Design review of the part built by this model. Coordinates are the model's own, in mm. A direction names the side the tool comes from. Give positions to 0.01 mm unless a question says otherwise; leave off trailing zeros. Write each loop counter-clockwise with the first axis right and the second up, starting at its lowest first coordinate (ties: lowest second). Pieces come first, ordered by that corner, then holes. Notation, with made-up numbers: M 39,25.25 L 91,25.25 A26 ccw 91,55.25 Z; hole C -27,7 d3. An arc over 180 degrees is marked long. Use a Markdown table: item, result. Add a question column.
```python
from build123d import *

# Parameters (mm, degrees)
F1_DEPTH       = 12.7
F3_D           = 3.302
F3_CBORE_D     = 6.5024
F3_CBORE_DEPTH = 0
F4_R           = 2.54


with BuildPart() as f1:
    # F0 (on Front) → F1 (new body)
    with BuildSketch(Plane.XZ):
        with BuildLine():
            Line((-50.8, 0), (0, 0))
            Line((0, 0), (25.4, 0))
            ThreePointArc((25.4, 0), (31.75, 6.35), (25.4, 12.7))
            Line((25.4, 12.7), (0, 12.7))
            Line((0, 12.7), (0, 6.35))
            Line((0, 6.35), (-50.8, 6.35))
            Line((-50.8, 6.35), (-50.8, 0))
        make_face()
    extrude(amount=F1_DEPTH)

    # F3 (through all)
    with Locations(Plane.XZ.offset(12.7)):
        with Locations((25.4, 6.35)):
            CounterBoreHole(F3_D / 2, F3_CBORE_D / 2, F3_CBORE_DEPTH)

    # F4
    f4_edges = [f1.edges().sort_by_distance(p)[0] for p in [
        (-50.8, -6.35, 6.35),
        (-50.8, -6.35, 0),
        (-50.8, 0, 3.175),
        (-50.8, -12.7, 3.175),
    ]]
    fillet(f4_edges, radius=F4_R)


solid = f1.part
```
(1) Add section C-C on z = 1.25. Give the boundary of the cut face in (x, y), then the cut area to 3 significant figures.
(2) Wall thickness on L1, parallel to X at y = -7.25, z = 6.5; L2, parallel to Z at x = 25.4, y = -2.5; L3, parallel to Z at x = 24, y = -1.5: over which ranges is each line inside the solid? List them lowest first.
(3) Add section A-A on y = -3.5. Give the boundary of the cut face in (x, z).
(4) For pin 1 (3 mm diameter, centred on y = -6.5, z = 11, fed in from -X); pin 2 (1.5 mm diameter, centred on y = -7.5, z = 2.5, fed in from +X); pin 3 (5 mm diameter, centred on x = -34.5, y = -8.5, fed in from +Z), all flat-tipped, find the tip position at first contact; note any pin that passes through.
(5) Machinability: for faces 1 (the flat face through (0, 0, 5)), 2 (the flat face through (-24, -6, 6.35)), which of the approach directions +Z, -Z, +X, -X, +Y, -Y give a long, thin tool a straight path to every point of the face, cutting with its end or side? Answer none if there is none.
(6) Add section B-B on x = -17. Give the boundary of the cut face in (y, z).
(7) The part is to be moulded in two halves that separate along Z. For faces 3 (the cylindrical face through (23.825, -6.261, 6.846)), 4 (the cylindrical face through (31.75, -6.26, 6.21)), 5 (the flat face through (13, -6, 12.7)), 6 (the flat face through (0, -6, 10)), say which applies: released by +Z, released by -Z, zero draft, split by the parting line, or undercut.
From the geometry:
| question | item | result |
|---|---|---|
| 1 | outline | M -50.45,-11.45 A2.54 ccw -48.26,-12.7 L 29.18,-12.7 L 29.18,0 L -48.26,0 A2.54 ccw -50.45,-1.25 Z |
| 1 | area | 1,010 mm^2 |
| 2 | L1 | x = 0 to 23.76, 27.04 to 31.75 |
| 2 | L2 | z = 0 to 4.7, 8 to 12.7 |
| 2 | L3 | z = 0 to 5.47, 7.23 to 12.7 |
| 3 | outline | M -50.8,2.54 A2.54 ccw -48.26,0 L 25.4,0 A6.35 ccw 25.4,12.7 L 0,12.7 L 0,6.35 L -48.26,6.35 A2.54 ccw -50.8,3.81 Z; hole C 25.4,6.35 d3.3 |
| 4 | pin 1 | stops at x = 0 |
| 4 | pin 2 | stops at x = 30.94 |
| 4 | pin 3 | stops at z = 6.35 |
| 5 | face 1 | +Z, -Z, +X, -X, +Y |
| 5 | face 2 | +Z, -X, +Y, -Y |
| 6 | outline | M -12.7,0 L 0,0 L 0,6.35 L -12.7,6.35 Z |
| 7 | face 3 | undercut |
| 7 | face 4 | split by the parting line |
| 7 | face 5 | released by +Z |
| 7 | face 6 | zero draft |
